Part model, mm, in its own coordinate system. Coordinates: 2 decimals unless noted, no trailing zeros. Loops run counter-clockwise (first coordinate to the right, second up) from the corner with the lowest first, then second, coordinate; pieces in that order, holes last. Notation, with made-up numbers: (17, -24.5) -> (72, -24.5) arc R15 ccw to (72, -12.5) -> close; hole circle Ø7 at (23.5, 18). An arc over 180 degrees is marked (long way). Use one line per item in the form item = value. Start each with the question number.
(1) Band-saw the part on C-C on x = -7.5. Give the cut face in (y, z) (3 decimals).
(2) Band-saw the part on D-D on y = 60. Give the cut face in (x, z) (3 decimals), then the cut area to 3 significant figures.
(3) Band-saw the part on A-A on y = 19. Give the cut face in (x, z), then the cut area to 3 significant figures.
(4) Pin check, flat tips, straight feed: P1, Ø2, axis at y = 47.5, z = 3, coming from the -X side; P2, Ø2, axis at x = 30.5, z = 3.5, coming from the +Y side. Stop position of each tip, or through.
(5) Band-saw the part on B-B on x = 7.5. Give the cut face in (y, z) (3 decimals), then the cut area to 3 significant figures.
(6) Drill centre lines: L1, parallel to X at y = 70.5, z = 1.05; L2, parallel to Y at x = -20, z = 2.15 (3 decimals); L3, parallel to X at y = 42, z = 3.1. Where is each one in solid material? Low to high. Write a range as [from, to].
```python
from build123d import *

# Parameters (mm, degrees)
EXTRUDE_1_DEPTH          = 4
EXTRUDE_2_DEPTH          = 4
CUT_EXTRUDE_2_DEPTH      = 4
CUT_EXTRUDE_3_DEPTH      = 4
SKETCH_8_R               = 1.525
CUT_EXTRUDE_4_DEPTH      = 10
SKETCH_9_R               = 2.025
CUT_EXTRUDE_5_DEPTH      = 10
CUT_EXTRUDE_6_DEPTH      = 1
CUT_EXTRUDE_6_DEPTH_BACK = 5
SKETCH_11_W              = 30
SKETCH_11_H              = 10
SKETCH_11_R              = 2.025
EXTRUDE_3_DEPTH          = 4
FILLET_2_R               = 3
EXTRUDE_4_DEPTH          = 4
FILLET_3_R               = 1


with BuildPart() as part:
    # 草图1 → 凸台-拉伸1 (new body)
    with BuildSketch(Plane.XY):
        Polygon((-45, 0), (45, 0), (45, 30), (15, 30), (15, 65), (-15, 65), (-15, 30), (-45, 30), align=None)
    extrude(amount=EXTRUDE_1_DEPTH)

    # 草图4 → 凸台-拉伸2 (add)
    with BuildSketch(Plane.XY.offset(4)):
        Polygon((-45, 30), (-15, 65), (-15, 30), align=None)
        Polygon((15, 65), (45, 30), (15, 30), align=None)
    extrude(amount=-EXTRUDE_2_DEPTH)

    # 草图5 → 切除-拉伸2 (cut)
    with BuildSketch(Plane.XY.offset(4)):
        Polygon((-38.414611102, 30), (-15, 30), (-15, 57.317046286), align=None)
        Polygon((15, 57.317046286), (38.414611102, 30), (15, 30), align=None)
    extrude(amount=-CUT_EXTRUDE_2_DEPTH, mode=Mode.SUBTRACT)

    # 草图6 → 切除-拉伸3 (cut)
    with BuildSketch(Plane.XY.offset(4)):
        Polygon((0, 54.050827988), (-9, 48.854675566), (-9, 38.46237072), (0, 33.266218297), (9, 38.46237072), (9, 48.854675566), align=None)
    extrude(amount=-CUT_EXTRUDE_3_DEPTH, mode=Mode.SUBTRACT)

    # 草图8 → 切除-拉伸4 (cut)
    with BuildSketch(Plane(origin=(0, 0, 0), x_dir=(-1, 0, 0), z_dir=(0, 0, -1))):
        with Locations((20.000000001, 14.999999905)):
            Circle(SKETCH_8_R)
        with Locations((-9.999999999, 14.999999905)):
            Circle(SKETCH_8_R)
        with Locations((-39.999999999, 14.999999905)):
            Circle(SKETCH_8_R)
    extrude(amount=-CUT_EXTRUDE_4_DEPTH, mode=Mode.SUBTRACT)

    # 草图9 → 切除-拉伸5 (cut)
    with BuildSketch(Plane(origin=(0, 0, 0), x_dir=(-1, 0, 0), z_dir=(0, 0, -1))):
        with Locations((-7.5, 60)):
            Circle(SKETCH_9_R)
        with Locations((7.5, 60)):
            Circle(SKETCH_9_R)
    extrude(amount=-CUT_EXTRUDE_5_DEPTH, mode=Mode.SUBTRACT)

    # 草图10 → 切除-拉伸6 (cut, two sides)
    with BuildSketch(Plane.XY.offset(4)) as cut_extrude_6_sk:
        with BuildLine():
            Line((-10.000000001, 19.999999905), (-1e-09, 19.999999905))
            ThreePointArc((-1e-09, 19.999999905), (4.999999999, 14.999999905), (-1e-09, 9.999999905))
            Line((-1e-09, 9.999999905), (-10.000000001, 9.999999905))
            ThreePointArc((-10.000000001, 9.999999905), (-15.000000001, 14.999999905), (-10.000000001, 19.999999905))
        make_face()
        with BuildLine():
            Line((19.999999999, 19.999999905), (29.999999999, 19.999999905))
            ThreePointArc((29.999999999, 19.999999905), (34.999999999, 14.999999905), (29.999999999, 9.999999905))
            Line((29.999999999, 9.999999905), (19.999999999, 9.999999905))
            ThreePointArc((19.999999999, 9.999999905), (14.999999999, 14.999999905), (19.999999999, 19.999999905))
        make_face()
        with BuildLine():
            Line((-36, 19.999999905), (-29, 19.999999905))
            ThreePointArc((-29, 19.999999905), (-24, 14.999999905), (-29, 9.999999905))
            Line((-29, 9.999999905), (-36, 9.999999905))
            ThreePointArc((-36, 9.999999905), (-41, 14.999999905), (-36, 19.999999905))
        make_face()
    extrude(amount=CUT_EXTRUDE_6_DEPTH, mode=Mode.SUBTRACT)
    extrude(cut_extrude_6_sk.sketch, amount=-CUT_EXTRUDE_6_DEPTH_BACK, mode=Mode.SUBTRACT)

    # 草图11 → 凸台-拉伸3 (add)
    with BuildSketch(Plane.XY.offset(4)):
        with Locations((0, 70)):
            Rectangle(SKETCH_11_W, SKETCH_11_H)
        with Locations((7.5, 70)):
            Circle(SKETCH_11_R, mode=Mode.SUBTRACT)
        with Locations((-7.5, 70)):
            Circle(SKETCH_11_R, mode=Mode.SUBTRACT)
    extrude(amount=-EXTRUDE_3_DEPTH)

    # 圆角2
    fillet_2_edges = [part.edges().sort_by_distance(p)[0] for p in [
        (-45, 30, 2),
        (-15, 65, 2),
        (15, 65, 2),
        (45, 30, 2),
        (45, 0, 2),
        (-45, 0, 2),
        (15, 75, 2),
        (-15, 75, 2),
    ]]
    fillet(fillet_2_edges, radius=FILLET_2_R)

    # 草图13 → 凸台-拉伸4 (add)
    with BuildSketch(Plane.XY.offset(4)):
        Polygon((15, 33.037026409), (26.997186292, 43.320328945), (29.600351786, 40.283302536), (17.603165494, 30), (15, 30), align=None)
    extrude_4 = extrude(amount=-EXTRUDE_4_DEPTH)

    # 镜向1: 凸台-拉伸4 across plane
    add(extrude_4.mirror(Plane(origin=(0, 0, 0), x_dir=(0, 0, 1), z_dir=(1, 0, 0))))

    # 圆角3
    fillet_3_edges = [part.edges().sort_by_distance(p)[0] for p in [
        (15, 33.037026409, 2),
        (26.997186292, 43.320328945, 2),
        (29.600351786, 40.283302536, 2),
        (17.603165494, 30, 2),
        (-26.997186292, 43.320328945, 2),
        (-29.600351786, 40.283302536, 2),
        (-17.603165494, 30, 2),
        (-15, 33.037026409, 2),
        (-38.414611102, 30, 2),
        (-15, 57.317046286, 2),
        (15, 57.317046286, 2),
        (38.414611102, 30, 2),
        (0, 54.050827988, 2),
        (9, 48.854675566, 2),
        (9, 38.46237072, 2),
        (0, 33.266218297, 2),
        (-9, 38.46237072, 2),
        (-9, 48.854675566, 2),
    ]]
    fillet(fillet_3_edges, radius=FILLET_3_R)


solid = part.part
```
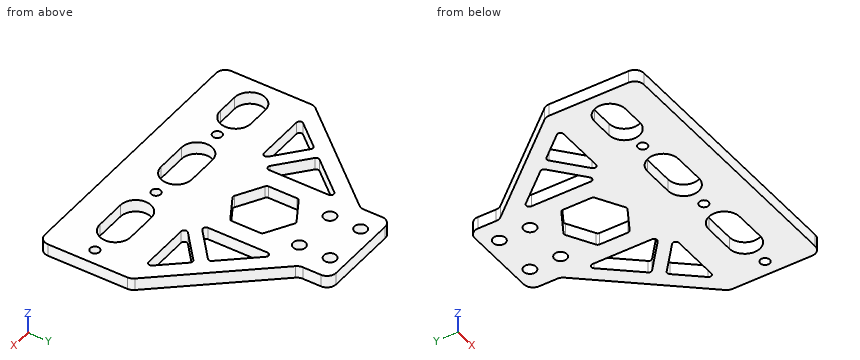
A:
q1.outline = (0, 0) -> (10, 0) -> (10, 4) -> (0, 4) -> close; (20, 0) -> (37.596, 0) -> (37.596, 4) -> (20, 4) -> close; (49.721, 0) -> (57.975, 0) -> (57.975, 4) -> (49.721, 4) -> close; (62.025, 0) -> (67.975, 0) -> (67.975, 4) -> (62.025, 4) -> close; (72.025, 0) -> (75, 0) -> (75, 4) -> (72.025, 4) -> close
q2.outline = (-19.286, 0) -> (-9.525, 0) -> (-9.525, 4) -> (-19.286, 4) -> close; (-5.475, 0) -> (5.475, 0) -> (5.475, 4) -> (-5.475, 4) -> close; (9.525, 0) -> (19.286, 0) -> (19.286, 4) -> (9.525, 4) -> close
q2.area = 122 mm²
q3.outline = (-45, 0) -> (-39, 0) -> (-39, 4) -> (-45, 4) -> close; (-26, 0) -> (-13, 0) -> (-13, 4) -> (-26, 4) -> close; (3, 0) -> (17, 0) -> (17, 4) -> (3, 4) -> close; (33, 0) -> (45, 0) -> (45, 4) -> (33, 4) -> close
q3.area = 180 mm²
q4.P1 = -30.86
q4.P2 = 48.08
q5.outline = (0, 0) -> (37.596, 0) -> (37.596, 4) -> (0, 4) -> close; (49.721, 0) -> (57.975, 0) -> (57.975, 4) -> (49.721, 4) -> close; (62.025, 0) -> (67.975, 0) -> (67.975, 4) -> (62.025, 4) -> close; (72.025, 0) -> (75, 0) -> (75, 4) -> (72.025, 4) -> close
q5.area = 219 mm²
q6.L1 = [-15, -9.46], [-5.54, 5.54], [9.46, 15]
q6.L2 = [0, 13.475], [16.525, 30.048], [32.054, 37.323], [51.484, 59.167]
q6.L3 = [-34.71, -25.46], [-15, -9], [9, 15], [25.46, 34.71]
